Geometry: final body of the model. Coordinates: model frame, mm. A direction names the side the tool comes from. Give positions to 0.01 mm unless a question says otherwise; leave off trailing zeros. Write each loop counter-clockwise with the first axis right and the second up, starting at its lowest first coordinate (ties: lowest second). Pieces come first, ordered by that corner, then holes. Notation, with made-up numbers: (80.25, 20) -> (135.25, 20) arc R35 ccw to (135.25, 59) -> close; hole circle Ø6 at (-18.75, 71). An arc over 180 degrees is marked (long way). Answer as a JSON object with one key per item and string values. Group by question number.
(1) Section query B-B on z = -6. Output: boundary loops of the cut face in (x, y), plus the area to 3 significant figures.
(2) Section query A-A on z = -30.1. Output: boundary loops of the cut face in (x, y), plus the area to 3 significant figures.
(3) Material intervals for probe 1 along X at (y, z) = (15.5, -30.1); probe 2 along Y at (x, z) = (1, -27); probe 3 along X at (y, z) = (10, 5), sorted ascending.
(4) Set-up query: faces 1 (the face through (15.5, 17.6, 4)), 2 (the face through (0, 12, 0)), 3 (the face through (-15.5, 17.6, 4)). Return all of +Z, -Z, +X, -X, +Y, -Y with unobstructed straight access to the full face (end or side cutting, diameter ignored); none if empty.
(5) Contact query for flat-ended pins moving along their axis: pin 1 Ø6 at (x, z) = (9, -30.1) entering from -Y; pin 2 Ø5 at (x, y) = (-5.5, 8.5) entering from -Z; pin 3 Ø1.7 at (x, y) = (15.5, 17) entering from +Z; pin 4 Ø2 at (x, y) = (-4, 13) entering from +Z. Output: stop coordinate, or through.
(6) Draft query along X for faces 4 (the face through (0, 14, -18)), 5 (the face through (-16, 14.3, -6.3)), 6 (the face through (-11.22, 16.03, -28.95)), 7 (the face through (16, 15, -8)). Return one class per face: +X half, -X half, draft (parallel to the pull), parting line (faces both ways), or undercut.
from build123d import *

# Parameters (mm, degrees)
BOSS_EXTRU_1_DEPTH      = 4
ESQUISSE2_W             = 32
ESQUISSE2_H             = 4
BOSS_EXTRU_2_DEPTH      = 36
BOSS_EXTRU_3_DEPTH      = 6
CONG_1_R                = 7
CHANFREIN1_SIZE         = 2
ESQUISSE4_R             = 2.5
ENL_V_MAT_EXTRU_1_DEPTH = 10


with BuildPart() as part:
    # Esquisse1 → Boss.-Extru.1 (new body)
    with BuildSketch(Plane.XY):
        with BuildLine():
            Line((-16, 18), (16, 18))
            Line((16, 18), (16, 0))
            Line((16, 0), (11.75, 0))
            ThreePointArc((11.75, 0), (0, 11.75), (-11.75, 0))
            Line((-11.75, 0), (-16, 0))
            Line((-16, 0), (-16, 18))
        make_face()
    extrude(amount=BOSS_EXTRU_1_DEPTH)

    # Esquisse2 → Boss.-Extru.2 (add)
    with BuildSketch(Plane(origin=(0, 0, 0), x_dir=(-1, 0, 0), z_dir=(0, 0, -1))):
        with Locations((0, 16)):
            Rectangle(ESQUISSE2_W, ESQUISSE2_H)
    extrude(amount=BOSS_EXTRU_2_DEPTH)

    # Esquisse3 → Boss.-Extru.3 (add)
    with BuildSketch(Plane.XY.offset(4)):
        with BuildLine():
            Line((-16, 0), (-11.75, 0))
            ThreePointArc((-11.75, 0), (0, 11.75), (11.75, 0))
            Line((11.75, 0), (16, 0))
            ThreePointArc((16, 0), (0, 16), (-16, 0))
        make_face()
    extrude(amount=BOSS_EXTRU_3_DEPTH)

    # Congé1
    # the kernel refuses this fillet: 7 mm, written as the material it adds along each edge
    with BuildSketch(Plane(origin=(0, 0, 4), x_dir=(1, 0, 0), z_dir=(0, -1, 0))) as cong_1_piece_1_section:
        with BuildLine():
            CenterArc((22.92820323, 7), CONG_1_R, 188.213210702, 81.786789298)
            Line((16, 6), (16, 0))
            Line((16, 0), (22.92820323, 0))
        make_face()
    cong_1_piece_1 = revolve(axis=Axis((0, 0, 4), (0, 0, 1)), revolution_arc=180, mode=Mode.PRIVATE)
    cong_1_piece_1 = split(cong_1_piece_1, bisect_by=Plane(origin=(0, 18, 4), z_dir=(0, -1, 0)), keep=Keep.TOP, mode=Mode.PRIVATE)
    cong_1_piece_1 = split(cong_1_piece_1, bisect_by=Plane(origin=(16, 0, 4), z_dir=(-1, 0, 0)), keep=Keep.TOP, mode=Mode.PRIVATE)
    cong_1_piece_1 = split(cong_1_piece_1, bisect_by=Plane(origin=(-16, 0, 4), z_dir=(1, 0, 0)), keep=Keep.TOP, mode=Mode.PRIVATE)
    add(cong_1_piece_1)

    # Chanfrein1
    chanfrein1_edges = [part.edges().sort_by_distance(p)[0] for p in [
        (0, 11.75, 10),
    ]]
    chamfer(chanfrein1_edges, length=CHANFREIN1_SIZE)

    # Esquisse4 → Enlèv. mat.-Extru.1 (cut)
    with BuildSketch(Plane(origin=(0, 18, 0), x_dir=(1, 0, 0), z_dir=(0, 1, 0))):
        with Locations(Location((9, 30.1, 0), (0, 0, 270))):
            Circle(ESQUISSE4_R)
        with Locations(Location((-9, 30.1, 0), (0, 0, 270))):
            Circle(ESQUISSE4_R)
    extrude(amount=-ENL_V_MAT_EXTRU_1_DEPTH, mode=Mode.SUBTRACT)


solid = part.part
Answer list:
{
 "1": {"outline": "(-16, 14) -> (16, 14) -> (16, 18) -> (-16, 18) -> close", "area": "128 mm2"},
 "2": {"outline": "(-16, 14) -> (-11.5, 14) -> (-11.5, 18) -> (-16, 18) -> close; (-6.5, 14) -> (6.5, 14) -> (6.5, 18) -> (-6.5, 18) -> close; (11.5, 14) -> (16, 14) -> (16, 18) -> (11.5, 18) -> close", "area": "88.0 mm2"},
 "3": {"probe 1": "-16 to -11.5, -6.5 to 6.5, 11.5 to 16", "probe 2": "14 to 18", "probe 3": "-16 to -6.17, 6.17 to 16"},
 "4": {"face 1": "+Z, +X, +Y", "face 2": "-Z, +X, -X, -Y", "face 3": "+Z, -X, +Y"},
 "5": {"pin 1": "y = 14", "pin 2": "z = 0", "pin 3": "z = 4.04", "pin 4": "z = 10"},
 "6": {"face 4": "draft", "face 5": "-X half", "face 6": "undercut", "face 7": "+X half"}
}
